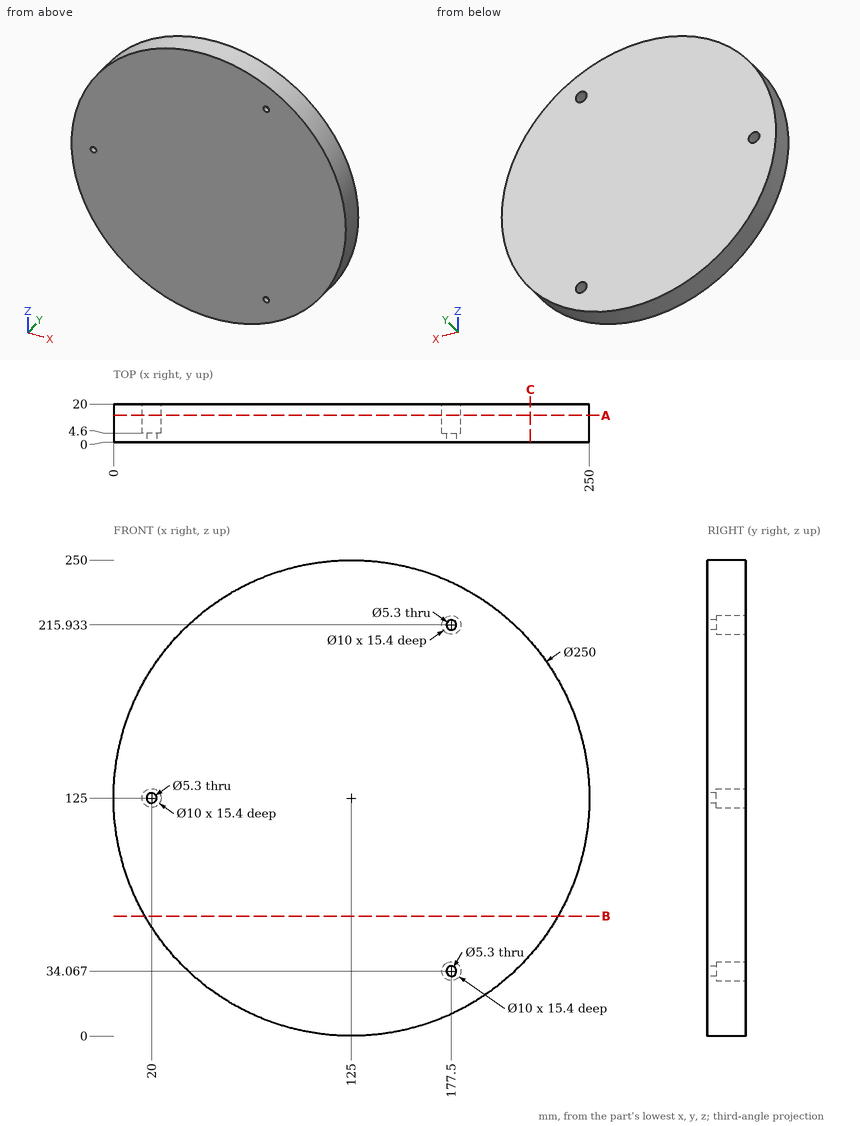
The drawing under review shows one solid part. Ordinate dimensions are in mm from its lowest x, y, z. Coordinates: 2 decimals unless noted, no trailing zeros. Loops run counter-clockwise (first coordinate to the right, second up) from the corner with the lowest first, then second, coordinate; pieces in that order, holes last. Notation, with made-up numbers: (72.5, 4) - (125.5, 4) arc R26 cw to (125.5, 18) - close; hole circle Ø7 at (5, 19.25). An arc over 180 degrees is marked (long way). Use CSV: the item, a comma, the result in double quotes. Start each with the question number.
1. To check wall thickness, follow probe 1 along Z at (x, y) = (177.5, 8); probe 2 along Z at (x, y) = (177.5, 1.6); probe 3 along X at (y, z) = (9.75, 125). State the ranges of each line that lie inside material, in increasing order.
2. Add section A-A on y = 14. Give the boundary of the cut face in (x, z).
3. Add section B-B on z = 63. Give the boundary of the cut face in (x, y).
4. Add section C-C on x = 219. Give the boundary of the cut face in (y, z) (1 decimal), plus the area to 3 significant figures.
5. Clearance check with flat-ended pins moving along their axes: pin 1 (1.5 mm diameter, centred on y = 2.5, z = 82.5, fed in from -X); pin 2 (6 mm diameter, centred on x = 20, z = 125, fed in from +Y); pin 3 (1 mm diameter, centred on y = 18, z = 214, fed in from -X); pin 4 (11 mm diameter, centred on x = 176, z = 34, fed in from +Y). State where each tip first meets the part, or that it passes through.
Resolved:
1,probe 1,"11.56 to 29.07, 39.07 to 210.93, 220.93 to 238.44"
1,probe 2,"11.56 to 31.42, 36.72 to 213.28, 218.58 to 238.44"
1,probe 3,"0 to 15, 25 to 250"
2,outline,"circle Ø250 at (125, 125); hole circle Ø10 at (20, 125); hole circle Ø10 at (177.5, 34.07); hole circle Ø10 at (177.5, 215.93)"
3,outline,"(16.46, 0) - (233.54, 0) - (233.54, 20) - (16.46, 20) - close"
4,outline,"(0, 42.6) - (20, 42.6) - (20, 207.4) - (0, 207.4) - close"
4,area,"3,300 mm2"
5,pin 1,"x = 7.18"
5,pin 2,"y = 4.6"
5,pin 3,"x = 36.72"
5,pin 4,"y = 20"
